from build123d import *

# Parameters (mm, degrees)
SKETCH016_R       = 1.85
EXTRUDE013_DEPTH  = 12
CYLINDER007_R     = 5
CYLINDER007_DEPTH = 1
EXTRUDE012_DEPTH  = 15


with BuildPart() as extrude013:
    # Sketch016 → Extrude013 (new body)
    with BuildSketch(Plane.XZ):
        Polygon((11.75, 36), (11.75, 19), (-13.25, 19), (-19.25, 25), (-19.25, 30), (-13.25, 36), align=None)
        with Locations((-14, 27.481564)):
            Circle(SKETCH016_R, mode=Mode.SUBTRACT)
    extrude(amount=-EXTRUDE013_DEPTH)


with BuildPart() as unprintable:
    # Cylinder007 → Cylinder007 (new body)
    with BuildSketch(Plane(origin=(-14, 18, 27.5), x_dir=(1, 0, 0), z_dir=(0, -1, 0))):
        Circle(CYLINDER007_R)
    extrude(amount=CYLINDER007_DEPTH)


with BuildPart() as body007:
    # Sketch015 → Extrude012 (new body)
    with BuildSketch(Plane.XY.offset(50)):
        with BuildLine():
            ThreePointArc((7.5, 0), (1.009178, 7.431794), (-7.228416, 2))
            Line((-7.228416, 2), (-21.228416, 2))
            Line((-21.228416, 4), (-21.228416, 2))
            Line((-8.616844, 4), (-21.228416, 4))
            ThreePointArc((9.5, 0), (2.048168, 9.276584), (-8.616844, 4))
            Line((7.5, 0), (9.5, 0))
        make_face()
    extrude(amount=EXTRUDE012_DEPTH)


with BuildPart() as body007_1:
    # Extrude012 placement: moved
    add(body007.part.moved(Location((0, 0, -30))))

    # Fusion016: union unprintable
    add(unprintable.part)

    # Common001: intersect Extrude013
    add(extrude013.part, mode=Mode.INTERSECT)


with BuildPart() as body007_2:
    # Common001 placement: moved
    add(body007_1.part.moved(Location((1.5, 0, 0))))


with BuildPart() as body007_3:
    # Clone007 placement: moved
    add(body007_2.part.moved(Location((-1.5, 0, 0))))


with BuildPart() as part_mirroring008:
    # Part__Mirroring008: instance of Body007
    add(body007_3.part.mirror(Plane(origin=(0, 0, 0), x_dir=(1, 0, 0), z_dir=(0, 1, 0))))


with BuildPart() as part_mirroring008_1:
    # Part__Mirroring008 placement: moved
    add(part_mirroring008.part.moved(Location((1.5, 0, 0))))


solid = part_mirroring008_1.part
The model under review builds one solid part; all positions refer to its coordinate system, in mm. A direction names the side the tool comes from. Round coordinates to 2 decimals unless told otherwise and drop trailing zeros. Loops run counter-clockwise (first coordinate to the right, second up) from the corner with the lowest first, then second, coordinate; pieces in that order, holes last. Notation, with made-up numbers: (-26.5, 53) -> (4.5, 53) arc R28 ccw to (4.5, 81) -> close; hole circle Ø4 at (-20.75, 29.5). An arc over 180 degrees is marked (long way). Write item = value, one per line. Start each with the question number.
Item 1: Insertion check: pin 1 (1.5 mm diameter, centred on x = 6, z = 32.5, fed in from -Y); pin 2 (5.5 mm diameter, centred on x = -14, z = 24.5, fed in from -Y); pin 3 (5 mm diameter, centred on y = -7, z = 33, fed in from -X). Each pin has a flat end and moves straight along its axis. Give the tip position at first contact, or say it passes through.
Item 2: For faces 1 (the flat face through (-15.215, -2.986, 22.465)), 2 (the flat face through (-10, -4, 27)), 3 (the flat face through (-10, -2, 27)), list the 3-axis set-ups (+Z, -Z, +X, -X, +Y, -Y) from which the entire face can be reached by the end or side of a thin tool; tool diameter is ignored.
Item 3: Take a section at C-C on z = 24. Give the boundary of the cut face in (x, y), plus the area to 3 significant figures.
Item 4: Take a section at A-A on x = -11.75. Give the boundary of the cut face in (y, z), plus the area to 3 significant figures.
Item 5: To check wall thickness, follow L1, parallel to Z at x = -12.5, y = -3.2; L2, parallel to X at y = -3.25, z = 28.75; L3, parallel to Y at x = -11.25, z = 30.75. State the ranges of each line that lie inside material, in increasing order.
Item 6: Take a section at D-D on x = -8.5. Give the boundary of the cut face in (y, z).
Item 7: Mouldability with a two-part tool opening along X and no side actions: class faces 4 (the flat face through (10, 0, 27)), 5 (the cylindrical face through (-12.901, -2.986, 25.676)), 6 (the flat face through (-15.28, -2.99, 32.47)) as released by +X, released by -X, zero draft, split by the parting line, or undercut.
Item 8: Take a section at B-B on y = -5.5. Give the boundary of the cut face in (x, z), plus the area to 3 significant figures.
Result:
q1.pin_1 = -8.73
q1.pin_2 = -4
q1.pin_3 = -6.87
q2.face_1 = -Z, -X, +Y, -Y
q2.face_2 = +Z, -Z, -X, -Y
q2.face_3 = +Z, -Z, -X, +Y
q3.outline = (-16.75, -4) -> (-7.12, -4) arc R9.5 ccw to (11, 0) -> (9, 0) arc R7.5 cw to (-5.73, -2) -> (-16.75, -2) -> close
q3.area = 67.9 mm²
q4.outline = (-4, 20) -> (-2, 20) -> (-2, 25.79) -> (-4, 25.79) -> close; (-4, 29.17) -> (-2, 29.17) -> (-2, 35) -> (-4, 35) -> close
q4.area = 23.2 mm²
q5.L1 = 20 to 25.63, 29.33 to 35
q5.L2 = -17.75 to -13.85, -11.15 to -5.26, 8.26 to 10.43
q5.L3 = -4 to -2
q6.outline = (-4, 20) -> (-2, 20) -> (-2, 35) -> (-4, 35) -> close
q7.face_4 = zero draft
q7.face_5 = undercut
q7.face_6 = released by -X
q8.outline = (-6.25, 20) -> (-3.6, 20) -> (-3.6, 35) -> (-6.25, 35) -> close; (6.6, 20) -> (9.25, 20) -> (9.25, 35) -> (6.6, 35) -> close
q8.area = 79.4 mm²
